Check sheet for the drawn part. Datum: minimum x, y, z corner. Units: mm. A direction names the side the tool comes from. Round coordinates to 2 decimals unless told otherwise and drop trailing zeros. Loops run counter-clockwise (first coordinate to the right, second up) from the corner with the lowest first, then second, coordinate; pieces in that order, holes last.
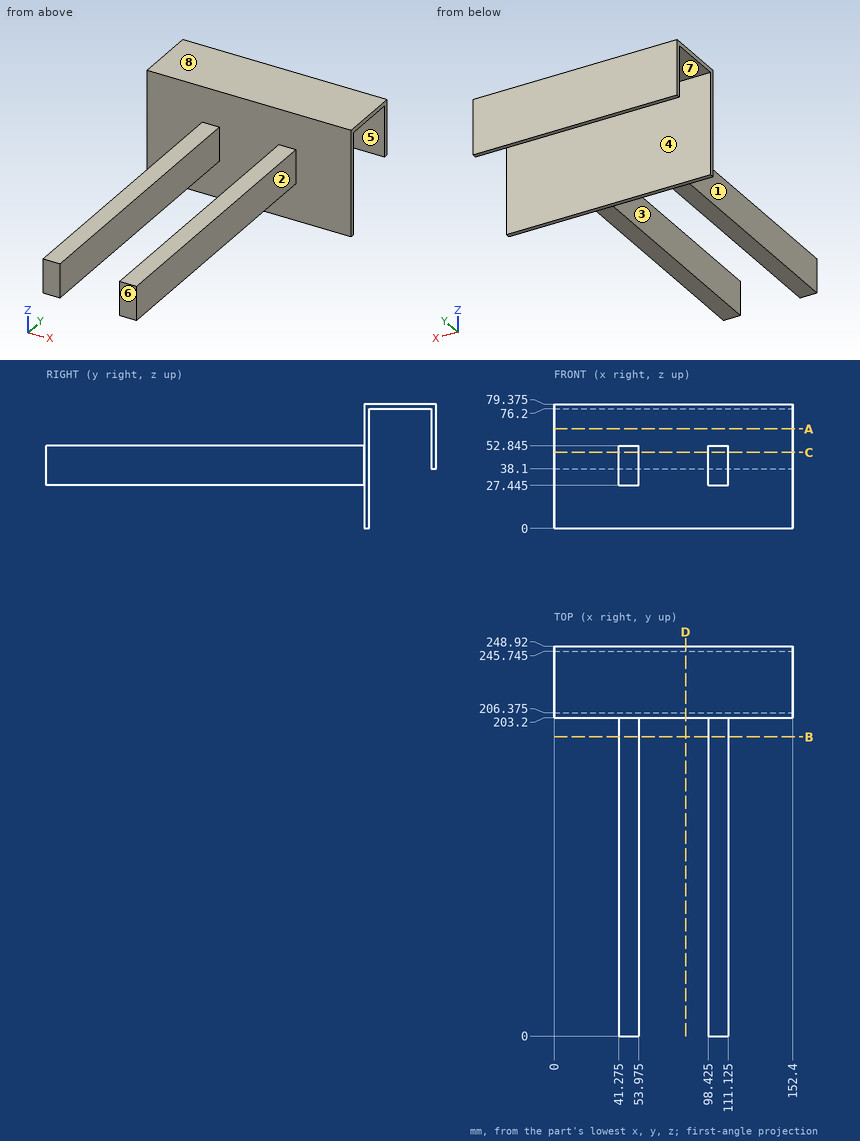
1. Gauge pin test, flat ends, axial feed: P1, Ø10, axis at x = 102, z = 17.5, coming from the -Y side; P2, Ø6.5, axis at x = 50, y = 135.5, coming from the -Z side (3 decimals); P3, Ø1.6, axis at x = 84.5, y = 248, coming from the -Z side; P4, Ø10, axis at y = 172, z = 62.5, coming from the +X side. Record the tip position at first contact, or that the pin passes through.
2. Section check B-B (y = 191). Enter the section's corners in (x, z) (3 decimals), then the cut area to 3 significant figures.
3. Scan lines: L1, parallel to X at y = 21, z = 45.5 (3 decimals); L2, parallel to Y at x = 20, z = 70.5 (3 decimals); L3, parallel to Y at x = 30.5, z = 19.5 (3 decimals). Record each from-to range of solid material in increasing order.
4. Tool access check on the marked faces 1, 2, 3 and 4. Record the directions out of +Z, -Z, +X, -X, +Y, -Y that give a thin tool (end or side, any length) a straight path to the whole face; none if there is none.
5. Section check D-D (x = 84). Enter the section's corners in (y, z) (3 decimals).
6. Section check C-C (z = 48.5). Enter the section's corners in (x, y) (3 decimals).
7. Section check A-A (z = 63.5). Enter the section's corners in (x, y) (3 decimals), then the cut area to 3 significant figures.
8. Release check for a two-part mould opening along Y. For the marked faces 5, 6, 7 and 8 record: released by +Y, released by -Y, zero draft, split by the parting line, or undercut.
Taken from the geometry:
1. P1: stops at y = 203.2
1. P2: stops at z = 27.445
1. P3: stops at z = 38.1
1. P4: passes through
2. outline: (41.275, 27.445) - (53.975, 27.445) - (53.975, 52.845) - (41.275, 52.845) - close; (98.425, 27.445) - (111.125, 27.445) - (111.125, 52.845) - (98.425, 52.845) - close
2. area: 645 mm2
3. L1: x = 41.275 to 53.975, 98.425 to 111.125
3. L2: y = 203.2 to 206.375, 245.745 to 248.92
3. L3: y = 203.2 to 206.375
4. face 1: +Z, -Z, -X, -Y
4. face 2: +Z, -Z, +X, -Y
4. face 3: +Z, -Z, -Y
4. face 4: -Z, +X, -X
5. outline: (203.2, 0) - (206.375, 0) - (206.375, 76.2) - (245.745, 76.2) - (245.745, 38.1) - (248.92, 38.1) - (248.92, 79.375) - (203.2, 79.375) - close
6. outline: (0, 203.2) - (41.275, 203.2) - (41.275, 0) - (53.975, 0) - (53.975, 203.2) - (98.425, 203.2) - (98.425, 0) - (111.125, 0) - (111.125, 203.2) - (152.4, 203.2) - (152.4, 206.375) - (0, 206.375) - close; (0, 245.745) - (152.4, 245.745) - (152.4, 248.92) - (0, 248.92) - close
7. outline: (0, 203.2) - (152.4, 203.2) - (152.4, 206.375) - (0, 206.375) - close; (0, 245.745) - (152.4, 245.745) - (152.4, 248.92) - (0, 248.92) - close
7. area: 968 mm2
8. face 5: undercut
8. face 6: released by -Y
8. face 7: undercut
8. face 8: zero draft
